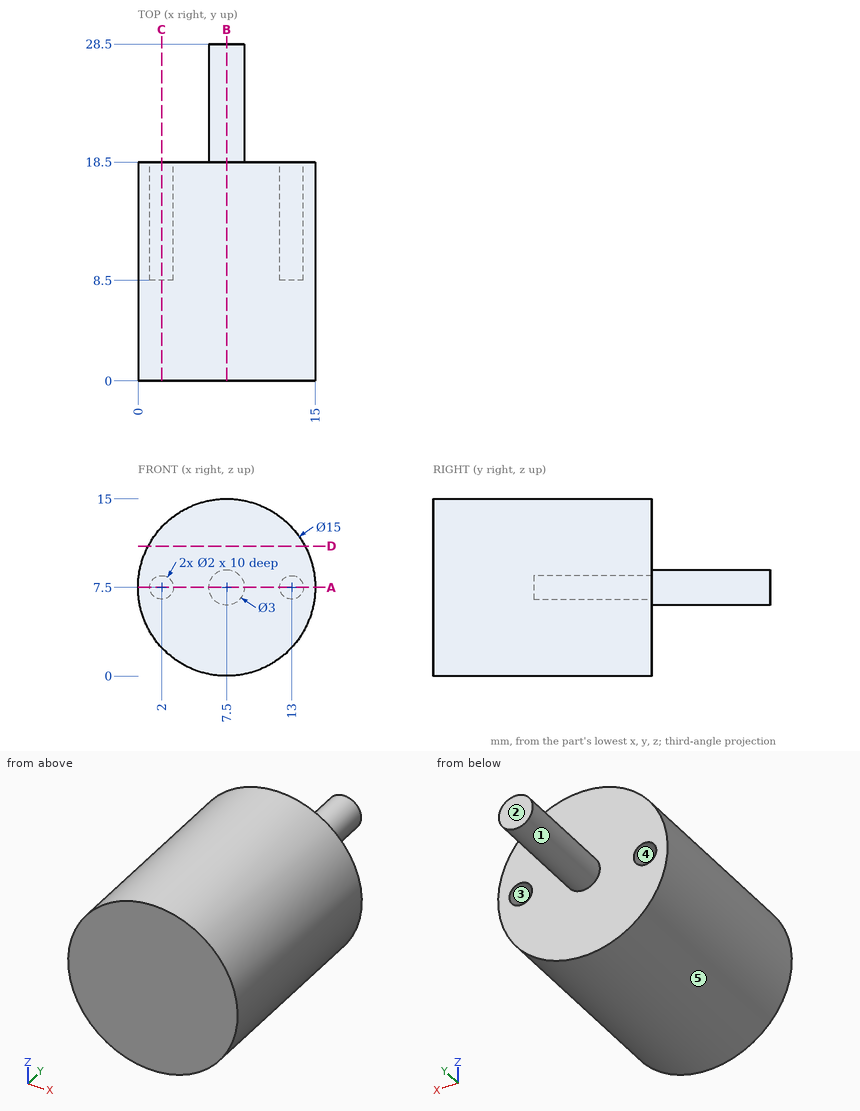
The figure shows three views and two pictorial views of one solid part (mm, origin at its lowest corner). Answer the questions. A direction names the side the tool comes from. Round coordinates to 2 decimals unless told otherwise and drop trailing zeros. Loops run counter-clockwise (first coordinate to the right, second up) from the corner with the lowest first, then second, coordinate; pieces in that order, holes last. Notation, with made-up numbers: (14.25, -7) - (18.25, -7) arc R34 cw to (18.25, 23) - close; hole circle Ø3 at (87, -2.75). An arc over 180 degrees is marked (long way). One line per question, with ' | ' between items. Start each with the question number.
Q1. Flat-ended cylindrical pins translate along their axes: pin 1 (1 mm diameter, centred on y = 10.5, z = 3, fed in from +X); pin 2 (0.6 mm diameter, centred on x = 13, z = 8, fed in from +Y); pin 3 (1.5 mm diameter, centred on x = 12, z = 6.5, fed in from +Y); pin 4 (6 mm diameter, centred on x = 5, z = 4, fed in from +Y). Find the tip coordinate at first contact, or state that the pin passes through.
Q2. For the marked faces 4 and 5, determine the directions among +Z, -Z, +X, -X, +Y, -Y from which every point of the face is accessible in a straight line to the end or side of a thin tool.
Q3. Section A-A on z = 7.5 is taken. Give the vertices of the cut face in (x, y).
Q4. Section B-B on x = 7.5 is taken. Give the vertices of the cut face in (y, z).
Q5. Section D-D on z = 11 is taken. Give the vertices of the cut face in (x, y), plus the area to 3 significant figures.
Q6. Section C-C on x = 2 is taken. Give the vertices of the cut face in (y, z), plus the area to 3 significant figures.
Q7. Find the intervals of material crossed by L1, parallel to X at y = 15.25, z = 7.5; L2, parallel to X at y = 11, z = 1.5; L3, parallel to Y at x = 7.25, z = 2, in increasing order.
Q8. For a pull along X with two mould halves and no side action, classify the marked faces 1, 2 and 3 as +X half, -X half, draft (parallel to the pull), parting line (faces both ways), or undercut.
Established:
1) pin 1: x = 13.84 | pin 2: y = 8.5 | pin 3: y = 18.5 | pin 4: y = 28.5
2) face 4: +Y | face 5: +Y, -Y
3) outline: (0, 0) - (15, 0) - (15, 18.5) - (14, 18.5) - (14, 8.5) - (12, 8.5) - (12, 18.5) - (9, 18.5) - (9, 28.5) - (6, 28.5) - (6, 18.5) - (3, 18.5) - (3, 8.5) - (1, 8.5) - (1, 18.5) - (0, 18.5) - close
4) outline: (0, 0) - (18.5, 0) - (18.5, 6) - (28.5, 6) - (28.5, 9) - (18.5, 9) - (18.5, 15) - (0, 15) - close
5) outline: (0.87, 0) - (14.13, 0) - (14.13, 18.5) - (0.87, 18.5) - close | area: 245 mm²
6) outline: (0, 2.4) - (18.5, 2.4) - (18.5, 6.5) - (8.5, 6.5) - (8.5, 8.5) - (18.5, 8.5) - (18.5, 12.6) - (0, 12.6) - close | area: 169 mm²
7) L1: 0 to 1, 3 to 12, 14 to 15 | L2: 3 to 12 | L3: 0 to 18.5
8) face 1: parting line | face 2: draft | face 3: undercut
